from build123d import *

# Parameters (mm, degrees)
F0_W     = 101.6
F0_H     = 76.2
F1_DEPTH = 50.8
F2_W     = 98.425
F2_H     = 98.425
F3_DEPTH = 73.025
F4_R     = 9.525
F5_DEPTH = 5.08


with BuildPart() as f1:
    # F0 (on Front) → F1 (new body, symmetric)
    with BuildSketch(Plane.XZ):
        Rectangle(F0_W, F0_H)
    extrude(amount=F1_DEPTH, both=True)

    # F2 (on face) → F3 (cut)
    with BuildSketch(Plane.XY.offset(38.1)):
        Rectangle(F2_W, F2_H)
    extrude(amount=-F3_DEPTH, mode=Mode.SUBTRACT)

    # F4 (on face) → F5 (join)
    with BuildSketch(Plane.YZ.offset(50.8)):
        with Locations((0, 26.531227)):
            Circle(F4_R)
    extrude(amount=F5_DEPTH)


solid = f1.part
Geometry check sheet. Reference: the model listing, model coordinates, mm. A direction names the side the tool comes from. Give positions to 0.01 mm unless a question says otherwise; leave off trailing zeros. Write each loop counter-clockwise with the first axis right and the second up, starting at its lowest first coordinate (ties: lowest second). Pieces come first, ordered by that corner, then holes.
1) Cross-section at C-C (y = -12). Record the boundary of the cut face in (x, z) (1 decimal).
Values follow:
outline: (-50.8, -38.1) - (50.8, -38.1) - (50.8, 38.1) - (49.2, 38.1) - (49.2, -34.9) - (-49.2, -34.9) - (-49.2, 38.1) - (-50.8, 38.1) - close
2) Set-up check for faces 1 (the face through (-1, 1, -34.925)), 2 (the face through (-1, -50.8, 1)): record each of +Z, -Z, +X, -X, +Y, -Y from which the full face is reachable in a straight line by a thin tool's end or side.
Values follow:
face 1: +Z
face 2: +Z, -Z, +X, -X, -Y
3) Cross-section at A-A (y = 0). Record the boundary of the cut face in (x, z) (1 decimal), plus the area to 3 significant figures.
Values follow:
outline: (-50.8, -38.1) - (50.8, -38.1) - (50.8, 17) - (55.9, 17) - (55.9, 36.1) - (50.8, 36.1) - (50.8, 38.1) - (49.2, 38.1) - (49.2, -34.9) - (-49.2, -34.9) - (-49.2, 38.1) - (-50.8, 38.1) - close
area: 651 mm2
4) Cross-section at B-B (z = 7). Record the boundary of the cut face in (x, y), plus the area to 3 significant figures.
Values follow:
outline: (-50.8, -50.8) - (50.8, -50.8) - (50.8, 50.8) - (-50.8, 50.8) - close; hole (-49.21, -49.21) - (49.21, -49.21) - (49.21, 49.21) - (-49.21, 49.21) - close
area: 635 mm2
5) Release check for a two-part mould opening along Y. For faces 3 (the face through (49.212, -1, 2)), 4 (the face through (53.3, -2.06, 17.23)), 5 (the face through (-1, 50.8, 1)), 6 (the face through (-50.8, -1, -1)) record: released by +Y, released by -Y, zero draft, split by the parting line, or undercut.
Values follow:
face 3: undercut
face 4: split by the parting line
face 5: released by +Y
face 6: zero draft
6) Go/stop test with a flat-tipped pin: pin 1 Ø23 at (y, z) = (19.5, 18.5) entering from +X. Record where the tip stops, or that it passes through.
Values follow:
pin 1: stops at x = 50.8
7) Thickness scan on line 1 (X direction, y = 11.5, z = 8.5); line 2 (X direction, y = 5.5, z = 24.5). Record the ranges inside material, lowest first.
Values follow:
line 1: x = -50.8 to -49.21, 49.21 to 50.8
line 2: x = -50.8 to -49.21, 49.21 to 55.88
